from build123d import *

# Parameters (mm, degrees)
F0_R          = 20
F1_DEPTH      = 30
F2_W          = 11.0205635428
F2_H          = 81.4056694508
F3_DEPTH      = 12
F3_DEPTH_BACK = 12
F4_W          = 11.5908719599
F4_H          = 48.789491877
F5_DEPTH      = 12


with BuildPart() as f1:
    # F0 (on Top) → F1 (new body)
    with BuildSketch(Plane.XY):
        Circle(F0_R)
    extrude(amount=F1_DEPTH)

    # F2 (on Top) → F3 (cut, two sides)
    with BuildSketch(Plane.XY) as f3_sk:
        with Locations((-5.5102817714, 0.5468949676)):
            Rectangle(F2_W, F2_H)
    extrude(amount=-F3_DEPTH, mode=Mode.SUBTRACT)
    extrude(f3_sk.sketch, amount=F3_DEPTH_BACK, mode=Mode.SUBTRACT)

    # F4 (on Top) → F5 (cut)
    with BuildSketch(Plane.XY):
        with Locations((17.6695231348, -3.9880210534)):
            Rectangle(F4_W, F4_H)
    extrude(amount=F5_DEPTH, mode=Mode.SUBTRACT)


solid = f1.part
Could you check a few things on this model? Use its own coordinates, in mm. A direction names the side the tool comes from. Coordinates: 2 decimals unless noted, no trailing zeros. Loops run counter-clockwise (first coordinate to the right, second up) from the corner with the lowest first, then second, coordinate; pieces in that order, holes last. Notation, with made-up numbers: (26, -10) -> (48, -10) arc R24 ccw to (48, 24) -> close; hole circle Ø6 at (11.5, 64.25). An arc over 180 degrees is marked (long way). Answer in a Markdown table with one row per item.
(1) Imagine slicing it at D-D (y = 8). List the corners of the cut face in (x, z) for me, plus the area to 3 significant figures.
Results found:
| item | result |
|---|---|
| outline | (-18.33, 0) -> (-11.02, 0) -> (-11.02, 12) -> (0, 12) -> (0, 0) -> (11.87, 0) -> (11.87, 12) -> (18.33, 12) -> (18.33, 30) -> (-18.33, 30) -> close |
| area | 890 mm^2 |
(2) If I drill on probe 1 along Z at (x, y) = (-4, 17); probe 2 along X at (y, z) = (-16, 11.25); probe 3 along Y at (x, z) = (-0.5, 16), over which ranges is the centre line in solid material (lowest first)?
Results found:
| item | result |
|---|---|
| probe 1 | z = 12 to 30 |
| probe 2 | x = -12 to -11.02, 0 to 11.87 |
| probe 3 | y = -19.99 to 19.99 |
(3) Imagine slicing it at B-B (y = 0). List the corners of the cut face in (x, z) for me, plus the area to 3 significant figures.
Results found:
| item | result |
|---|---|
| outline | (-20, 0) -> (-11.02, 0) -> (-11.02, 12) -> (0, 12) -> (0, 0) -> (11.87, 0) -> (11.87, 12) -> (20, 12) -> (20, 30) -> (-20, 30) -> close |
| area | 970 mm^2 |
(4) Will these pins go through, and if not, where does the flat tip stop? pin 1 Ø9.5 at (y, z) = (6.5, 7) entering from +X; pin 2 Ø8 at (y, z) = (13.5, 21) entering from -X; pin 3 Ø2 at (x, z) = (-10.5, 9.5) entering from +Y.
Results found:
| item | result |
|---|---|
| pin 1 | stops at x = 11.87 |
| pin 2 | stops at x = -17.6 |
| pin 3 | stops at y = 16.69 |
(5) Imagine slicing it at C-C (z = 18.5). List the corners of the cut face in (x, y) for me.
Results found:
| item | result |
|---|---|
| outline | circle Ø40 at (0, 0) |
(6) For faces 5 (the face through (0, 0, 6)), 6 (the face through (6, 0, 0)), which set-ups out of +Z, -Z, +X, -X, +Y, -Y let a thin tool reach every point of the face, with its end or its side?
Results found:
| item | result |
|---|---|
| face 5 | -Z, +Y, -Y |
| face 6 | -Z, +X, -X, +Y, -Y |
(7) Thinking about a two-plate mould opening in X: for faces 1 (the face through (-19.98, 0.88, 18.12)), 2 (the face through (11.874, 0, 6)), 3 (the face through (15, 0, 12)), 4 (the face through (-11.021, 0, 6)), which applies, released by +X, released by -X, zero draft, split by the parting line, or undercut?
Results found:
| item | result |
|---|---|
| face 1 | split by the parting line |
| face 2 | released by +X |
| face 3 | zero draft |
| face 4 | undercut |
(8) Imagine slicing it at A-A (z = 8.75). List the corners of the cut face in (x, y) for me, plus the area to 3 significant figures.
Results found:
| item | result |
|---|---|
| outline | (-11.02, -16.69) -> (-11.02, 16.69) arc R20 ccw to start; (0, -20) arc R20 ccw to (11.87, -16.09) -> (11.87, 16.09) arc R20 ccw to (0, 20) -> close |
| area | 656 mm^2 |
